Could you check a few things on this model? Use its own coordinates, in mm. A direction names the side the tool comes from. Coordinates: 2 decimals unless noted, no trailing zeros. Order: outer loops, then holes, each group sorted by start corner. A loop starts at its lowest first (then second) coordinate and runs counter-clockwise, first axis right, second up. Notation, with made-up numbers: (16, 16.25) - (57, 16.25) arc R34 cw to (57, 48.25) - close; hole circle Ø10 at (87.25, 89.5). An arc over 180 degrees is marked (long way). One line per item, written item: value. Start each with the question number.
from build123d import *

# Parameters (mm, degrees)
BOSS_EXTRUDE1_DEPTH = 1
SKETCH2_R           = 2.5
BOSS_EXTRUDE2_DEPTH = 7.5
FILLET1_R           = 2.5
SKETCH3_W           = 0.5
SKETCH3_H           = 0.5
BOSS_EXTRUDE3_DEPTH = 26
SKETCH4_W           = 0.5
SKETCH4_H           = 0.5
BOSS_EXTRUDE4_DEPTH = 1


with BuildPart() as part:
    # Sketch1 → Boss-Extrude1 (new body)
    with BuildSketch(Plane(origin=(0, 0, 0), x_dir=(1, 0, 0), z_dir=(0, 1, 0))):
        with BuildLine():
            Line((-2.5, 1.658312395), (-2.5, -1.658312395))
            ThreePointArc((-2.5, -1.658312395), (3, 0), (-2.5, 1.658312395))
        make_face()
    extrude(amount=BOSS_EXTRUDE1_DEPTH)

    # Sketch2 → Boss-Extrude2 (add)
    with BuildSketch(Plane(origin=(0, 1, 0), x_dir=(1, 0, 0), z_dir=(0, 1, 0))):
        with Locations(Location((0, 0, 0), (0, 0, 180))):
            Circle(SKETCH2_R)
    extrude(amount=BOSS_EXTRUDE2_DEPTH)

    # Fillet1
    fillet1_edges = [part.edges().sort_by_distance(p)[0] for p in [
        (2.5, 8.5, 0),
    ]]
    fillet(fillet1_edges, radius=FILLET1_R)

    # Sketch3 → Boss-Extrude3 (add)
    with BuildSketch(Plane(origin=(0, 0, 0), x_dir=(1, 0, 0), z_dir=(0, 1, 0))):
        with Locations((-1.4, 0)):
            Rectangle(SKETCH3_W, SKETCH3_H)
        with Locations((1.4, 0)):
            Rectangle(SKETCH3_W, SKETCH3_H)
    extrude(amount=-BOSS_EXTRUDE3_DEPTH)

    # Sketch4 → Boss-Extrude4 (add)
    with BuildSketch(Plane.XZ.offset(26)):
        with Locations((1.4, 0)):
            Rectangle(SKETCH4_W, SKETCH4_H)
    extrude(amount=BOSS_EXTRUDE4_DEPTH)


solid = part.part
Q1. I want a section at C-C on z = -0.8. Please give me the cut outline in (x, y), then the cut area to 3 significant figures.
Q2. I want a section at B-B on x = 0. Please give me the cut outline in (y, z).
Q3. I'm going to push flat-ended pins straight in: pin 1 (1.6 mm diameter, centred on x = 0, z = -0.5, fed in from -Y); pin 2 (0.6 mm diameter, centred on x = -1.5, z = 0, fed in from -Y); pin 3 (0.6 mm diameter, centred on y = -14, z = 0, fed in from +X). Where does each tip first touch, or does it pass through?
Q4. I want a section at A-A on y = -23. Please give me the cut outline in (x, z), then the cut area to 3 significant figures.
Q5. Which directions (+Z, -Z, +X, -X, +Y, -Y) give clear straight access to the entire face, cutting with the end or side of a thin tool? Please do faces 1 (the flat face through (-2.5, 0.5, 0)), 2 (the flat face through (2, 1, 2)).
Q6. If I drill on L1, parallel to Z at x = 1.55, y = -3; L2, parallel to X at y = -2, z = 0.2; L3, parallel to Y at x = 1, z = -2.35, over which ranges is the centre line in solid material (lowest first)?
Q7. I want a section at D-D on y = 0.5. Please give me the cut outline in (x, z).
Values follow:
1. outline: (-2.5, 0) - (2.89, 0) - (2.89, 1) - (2.37, 1) - (2.37, 6) arc R2.37 ccw to (-2.37, 6) - (-2.37, 1) - (-2.5, 1) - close
1. area: 37.9 mm^2
2. outline: (0, -3) - (1, -3) - (1, -2.5) - (6, -2.5) arc R2.5 ccw to (6, 2.5) - (1, 2.5) - (1, 3) - (0, 3) - close
3. pin 1: stops at y = 0
3. pin 2: stops at y = -26
3. pin 3: stops at x = 1.65
4. outline: (-1.65, -0.25) - (-1.15, -0.25) - (-1.15, 0.25) - (-1.65, 0.25) - close; (1.15, -0.25) - (1.65, -0.25) - (1.65, 0.25) - (1.15, 0.25) - close
4. area: 0.500 mm^2
5. face 1: +Z, -Z, -X, +Y, -Y
5. face 2: +Y
6. L1: z = -0.25 to 0.25
6. L2: x = -1.65 to -1.15, 1.15 to 1.65
6. L3: y = 0 to 1
7. outline: (-2.5, -1.66) arc R3 ccw (long way) to (-2.5, 1.66) - close
